```python
from build123d import *

# Parameters (mm, degrees)
BOSS_EXTRUDE1_DEPTH = 3.175
BOSS_EXTRUDE3_START = -3.175
BOSS_EXTRUDE3_DEPTH = 3.175


# Read off the part's stored shape, not the designer's step: Boss-Extrude3
with BuildPart() as part:
    # Sketch3 → Boss-Extrude1 (new body)
    with BuildSketch(Plane.XZ):
        with BuildLine():
            ThreePointArc((65.405, 0), (-28.808992359, 58.718446712), (-40.025960454, -51.727521831))
            Line((-40.025960454, -51.727521831), (-40.025960454, -33.675960454))
            ThreePointArc((-40.025960454, -33.675960454), (-33.675960454, -27.325960454), (-27.325960454, -33.675960454))
            Line((-27.325960454, -33.675960454), (-27.325960454, -53.995960454))
            ThreePointArc((-27.325960454, -53.995960454), (-27.817666914, -56.446041432), (-29.21663661, -58.516682836))
            ThreePointArc((-29.21663661, -58.516682836), (0, -65.405), (29.21663661, -58.516682836))
            ThreePointArc((29.21663661, -58.516682836), (27.817666914, -56.446041432), (27.325960454, -53.995960454))
            Line((27.325960454, -53.995960454), (27.325960454, -33.675960454))
            ThreePointArc((27.325960454, -33.675960454), (33.675960454, -27.325960454), (40.025960454, -33.675960454))
            Line((40.025960454, -33.675960454), (40.025960454, -51.727521831))
            ThreePointArc((40.025960454, -51.727521831), (58.718446712, -28.808992359), (65.405, 0))
        make_face()
        with BuildLine():
            ThreePointArc((-5.8, 0), (0, 5.8), (5.8, 0))
            Line((5.8, 0), (5.8, -20.32))
            ThreePointArc((5.8, -20.32), (0, -26.12), (-5.8, -20.32))
            Line((-5.8, -20.32), (-5.8, 0))
        make_face(mode=Mode.SUBTRACT)
        with BuildLine():
            ThreePointArc((-27.305960454, 13.355960454), (-33.675960454, 6.985960454), (-40.045960454, 13.355960454))
            Line((-40.045960454, 13.355960454), (-40.045960454, 33.675960454))
            ThreePointArc((-40.045960454, 33.675960454), (-33.675960454, 40.045960454), (-27.305960454, 33.675960454))
            Line((-27.305960454, 33.675960454), (-27.305960454, 13.355960454))
        make_face(mode=Mode.SUBTRACT)
        with BuildLine():
            ThreePointArc((40.025960454, 13.355960454), (33.675960454, 7.005960454), (27.325960454, 13.355960454))
            Line((27.325960454, 13.355960454), (27.325960454, 33.675960454))
            ThreePointArc((27.325960454, 33.675960454), (33.675960454, 40.025960454), (40.025960454, 33.675960454))
            Line((40.025960454, 33.675960454), (40.025960454, 13.355960454))
        make_face(mode=Mode.SUBTRACT)
    extrude(amount=BOSS_EXTRUDE1_DEPTH)

    # Boss-Extrude3 outline → Boss-Extrude3 (add)
    with BuildSketch(Plane(origin=(0, 0, 0), x_dir=(1, 0, 0), z_dir=(0, 1, 0)).offset(BOSS_EXTRUDE3_START)):
        with BuildLine():
            Line((-4.952891864, -1.691319584), (-4.952891864, -1.246819584))
            ThreePointArc((-4.952891864, -1.246819584), (-4.879618202, -1.014425219), (-4.6863, -0.866086946))
            Line((-4.6863, -0.866086946), (-3.328347771, -0.371832755))
            ThreePointArc((-3.328347771, -0.371832755), (-3.253985597, -0.314772651), (-3.2258, -0.22537936))
            Line((-3.2258, -0.22537936), (-3.2258, 0.22537936))
            ThreePointArc((-3.2258, 0.22537936), (-3.253985597, 0.314772651), (-3.328347771, 0.371832755))
            Line((-3.328347771, 0.371832755), (-4.6863, 0.866086946))
            ThreePointArc((-4.6863, 0.866086946), (-4.952891864, 1.246819585), (-4.6863, 1.627552223))
            Line((-4.6863, 1.627552223), (-3.328347771, 2.121806414))
            ThreePointArc((-3.328347771, 2.121806414), (-3.253985597, 2.178866518), (-3.2258, 2.268259809))
            Line((-3.2258, 2.268259809), (-3.2258, 2.719018529))
            ThreePointArc((-3.2258, 2.719018529), (-3.253985597, 2.80841182), (-3.328347771, 2.865471924))
            Line((-3.328347771, 2.865471924), (-4.6863, 3.359726115))
            ThreePointArc((-4.6863, 3.359726115), (-4.952891864, 3.740458754), (-4.6863, 4.121191392))
            Line((-4.6863, 4.121191392), (-3.328347771, 4.615445582))
            ThreePointArc((-3.328347771, 4.615445582), (-3.253985597, 4.672505686), (-3.2258, 4.761898978))
            Line((-3.2258, 4.761898978), (-3.2258, 5.212657697))
            ThreePointArc((-3.2258, 5.212657697), (-3.253985597, 5.302050989), (-3.328347771, 5.359111093))
            Line((-3.328347771, 5.359111093), (-4.6863, 5.853365283))
            ThreePointArc((-4.6863, 5.853365283), (-4.952891864, 6.234097921), (-4.6863, 6.61483056))
            Line((-4.6863, 6.61483056), (-3.328347771, 7.109084751))
            ThreePointArc((-3.328347771, 7.109084751), (-3.253985597, 7.166144855), (-3.2258, 7.255538147))
            Line((-3.2258, 7.255538147), (-3.2258, 7.706296866))
            ThreePointArc((-3.2258, 7.706296866), (-3.253985597, 7.795690157), (-3.328347771, 7.852750261))
            Line((-3.328347771, 7.852750261), (-4.6863, 8.347004452))
            ThreePointArc((-4.6863, 8.347004452), (-4.952891864, 8.72773709), (-4.6863, 9.108469729))
            Line((-4.6863, 9.108469729), (-3.328347771, 9.60272392))
            ThreePointArc((-3.328347771, 9.60272392), (-3.253985597, 9.659784024), (-3.2258, 9.749177315))
            Line((-3.2258, 9.749177315), (-3.2258, 10.199936035))
            ThreePointArc((-3.2258, 10.199936035), (-3.253985597, 10.289329326), (-3.328347771, 10.34638943))
            Line((-3.328347771, 10.34638943), (-4.6863, 10.840643621))
            ThreePointArc((-4.6863, 10.840643621), (-4.952891864, 11.221376259), (-4.6863, 11.602108898))
            Line((-4.6863, 11.602108898), (-3.328347771, 12.096363089))
            ThreePointArc((-3.328347771, 12.096363089), (-3.253985597, 12.153423193), (-3.2258, 12.242816484))
            Line((-3.2258, 12.242816484), (-3.2258, 12.693575204))
            ThreePointArc((-3.2258, 12.693575204), (-3.253985597, 12.782968495), (-3.328347771, 12.840028599))
            Line((-3.328347771, 12.840028599), (-4.6863, 13.33428279))
            ThreePointArc((-4.6863, 13.33428279), (-4.952891864, 13.715015428), (-4.6863, 14.095748067))
            Line((-4.6863, 14.095748067), (-3.328347771, 14.590002258))
            ThreePointArc((-3.328347771, 14.590002258), (-3.253985597, 14.647062362), (-3.2258, 14.736455653))
            Line((-3.2258, 14.736455653), (-3.2258, 15.187214372))
            ThreePointArc((-3.2258, 15.187214372), (-3.253985597, 15.276607664), (-3.328347771, 15.333667768))
            Line((-3.328347771, 15.333667768), (-4.6863, 15.827921959))
            ThreePointArc((-4.6863, 15.827921959), (-4.952891864, 16.208654598), (-4.6863, 16.589387236))
            Line((-4.6863, 16.589387236), (-3.328347771, 17.083641426))
            ThreePointArc((-3.328347771, 17.083641426), (-3.253985597, 17.14070153), (-3.2258, 17.230094822))
            Line((-3.2258, 17.230094822), (-3.2258, 17.680853541))
            ThreePointArc((-3.2258, 17.680853541), (-3.253985597, 17.770246833), (-3.328347771, 17.827306937))
            Line((-3.328347771, 17.827306937), (-4.6863, 18.321561127))
            ThreePointArc((-4.6863, 18.321561127), (-4.952891864, 18.702293766), (-4.6863, 19.083026404))
            Line((-4.6863, 19.083026404), (-3.328347771, 19.577280595))
            ThreePointArc((-3.328347771, 19.577280595), (-3.253985597, 19.634340699), (-3.2258, 19.723733991))
            Line((-3.2258, 19.723733991), (-3.2258, 20.17449271))
            ThreePointArc((-3.2258, 20.17449271), (-3.253985597, 20.263886001), (-3.328347771, 20.320946105))
            Line((-3.328347771, 20.320946105), (-4.6863, 20.815200296))
            ThreePointArc((-4.6863, 20.815200296), (-4.879618202, 20.96353857), (-4.952891864, 21.195932935))
            Line((-4.952891864, 21.195932935), (-4.952891864, 21.640432935))
            ThreePointArc((-4.952891864, 21.640432935), (-4.26463583, 23.987869264), (-2.41779287, 25.592027849))
            ThreePointArc((-2.41779287, 25.592027849), (-4.881761908, 23.45183663), (-5.8, 20.32))
            Line((-5.8, 20.32), (-5.8, 0))
            ThreePointArc((-5.8, 0), (-5.240594871, -2.485189209), (-3.670287792, -4.490989593))
            Line((-3.670287792, -4.490989593), (-3.662076811, -4.493978146))
            ThreePointArc((-3.662076811, -4.493978146), (-4.614680156, -3.234133451), (-4.952891864, -1.691319584))
        make_face()
    extrude(amount=BOSS_EXTRUDE3_DEPTH)


solid = part.part
```
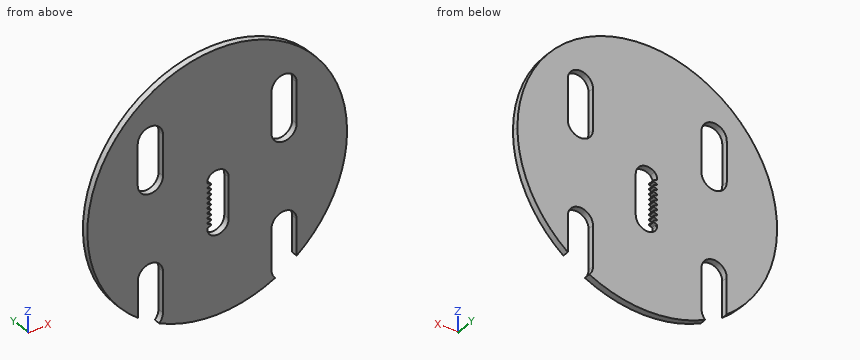
Work out the finished part from the listing and answer in its coordinate system (mm). Give positions to 0.01 mm unless a question says otherwise; leave off trailing zeros. Write each loop counter-clockwise with the first axis right and the second up, starting at its lowest first coordinate (ties: lowest second). Pieces come first, ordered by that corner, then holes.
(1) Flat-ended cylindrical pins translate along their axes: pin 1 Ø1 at (y, z) = (-2, -12.5) entering from -X; pin 2 Ø1 at (y, z) = (-1.5, 23) entering from -X; pin 3 Ø1 at (y, z) = (-1.5, -42) entering from +X; pin 4 Ø4 at (x, z) = (-50.5, 20.5) entering from +Y. Find the tip coordinate at first contact, or state that the pin passes through.
Final values:
pin 1: stops at x = -64.29
pin 2: stops at x = -61.41
pin 3: stops at x = 50.55
pin 4: stops at y = 0
(2) Straight lines are drawn through the part: line 1 (X direction, y = -1.6, z = 19.5); line 2 (X direction, y = -0.5, z = 8); line 3 (Z direction, x = -40.5, y = -0.35). For each, find the intervals that lie inside material, in ascending order.
Final values:
line 1: x = -62.43 to -40.05, -27.31 to 27.33, 40.03 to 62.43
line 2: x = -64.91 to -37.12, -30.23 to 30.26, 37.09 to 64.91
line 3: z = -51.36 to 51.36
(3) The part is cut by section A-A on x = 0. Write down the section's boundary in (y, z) (3 decimals).
Final values:
outline: (-3.175, -65.405) - (0, -65.405) - (0, -26.12) - (-3.175, -26.12) - close; (-3.175, 5.8) - (0, 5.8) - (0, 65.405) - (-3.175, 65.405) - close
(4) The part is cut by section D-D on z = 36.5. Write down the section's boundary in (x, y) (1 decimal), plus the area to 3 significant figures.
Final values:
outline: (-54.3, -3.2) - (-39.4, -3.2) - (-39.4, 0) - (-54.3, 0) - close; (-28, -3.2) - (28, -3.2) - (28, 0) - (-28, 0) - close; (39.4, -3.2) - (54.3, -3.2) - (54.3, 0) - (39.4, 0) - close
area: 272 mm2
(5) The part is cut by section C-C on y = -2.35. Count the separate pieces of the cut face and the enclosed holes in it, plus the area to 3 significant figures.
Final values:
separate pieces: 1
enclosed holes: 3
area: 11,700 mm2
(6) The part is cut by section B-B on z = -38.5. Write down the section's boundary in (x, y) (3 decimals).
Final values:
outline: (-52.873, -3.175) - (-40.026, -3.175) - (-40.026, 0) - (-52.873, 0) - close; (-27.326, -3.175) - (27.326, -3.175) - (27.326, 0) - (-27.326, 0) - close; (40.026, -3.175) - (52.873, -3.175) - (52.873, 0) - (40.026, 0) - close
